```python
from build123d import *

# Parameters (mm, degrees)
SKETCH1_W                                = 152.4
SKETCH1_H                                = 101.6
BOSS_EXTRUDE1_DEPTH                      = 12.7
CBORE_FOR_3_8_HEX_HEAD_BOLT1_D           = 10.0838
CBORE_FOR_3_8_HEX_HEAD_BOLT1_CBORE_D     = 15.24
CBORE_FOR_3_8_HEX_HEAD_BOLT1_CBORE_DEPTH = 11.176
TAP_DRILL_FOR_1_4_20_TAP1_D              = 5.1054


with BuildPart() as part:
    # Sketch1 → Boss-Extrude1 (new body)
    with BuildSketch(Plane(origin=(0, 0, 0), x_dir=(1, 0, 0), z_dir=(0, 1, 0))):
        Rectangle(SKETCH1_W, SKETCH1_H)
    extrude(amount=BOSS_EXTRUDE1_DEPTH)

    # CBORE for 3/8 Hex Head Bolt1 (through all)
    with Locations(Plane(origin=(0, 12.7, 0), x_dir=(1, 0, 0), z_dir=(0, 1, 0))):
        with Locations((-50.000000076, 0), (50.000000076, 0), (0, 0)):
            CounterBoreHole(CBORE_FOR_3_8_HEX_HEAD_BOLT1_D / 2, CBORE_FOR_3_8_HEX_HEAD_BOLT1_CBORE_D / 2, CBORE_FOR_3_8_HEX_HEAD_BOLT1_CBORE_DEPTH)

    # Tap Drill for 1/4-20 Tap1 (through all)
    with Locations(Plane.XZ):
        with Locations((-38.1, -38.1), (38.1, -38.1), (38.1, 38.1), (-38.1, 38.1)):
            Hole(TAP_DRILL_FOR_1_4_20_TAP1_D / 2)


solid = part.part
```
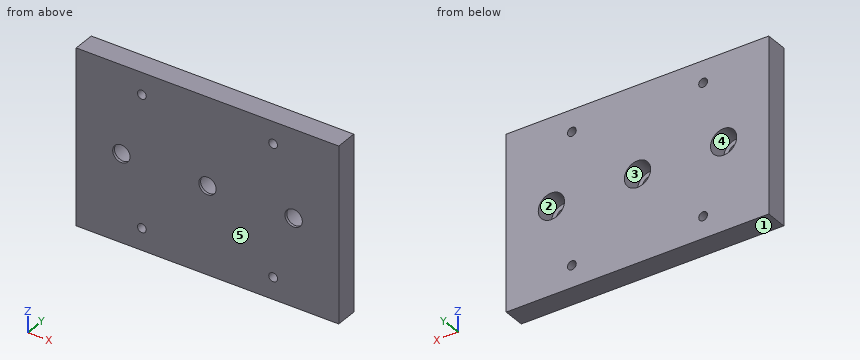
Geometry check sheet. Reference: the model listing, model coordinates, mm. Face numbers are marked on the shaded views. A direction names the side the tool comes from. Give positions to 0.01 mm unless a question says otherwise; leave off trailing zeros. Order: outer loops, then holes, each group sorted by start corner. A loop starts at its lowest first (then second) coordinate and runs counter-clockwise, first axis right, second up. Notation, with made-up numbers: (-2, 46) -> (46, 46) arc R12 cw to (46, 66) -> close; hole circle Ø4 at (21, -1). An arc over 180 degrees is marked (long way). Write each question's results on one line, items separated by ' | '. Start each with the question number.
(1) Sectioned sample at A-A (x = 38.1). Enter the section's corners in (y, z), plus the area to 3 significant figures.
(2) Sectioned sample at C-C (x = -50). Enter the section's corners in (y, z).
(3) Scan lines: line 1 (Z direction, x = -38.1, y = 4.75); line 2 (Z direction, x = -50, y = 0.95); line 3 (X direction, y = 6, z = -3). Record each from-to range of solid material in increasing order.
(4) Sectioned sample at B-B (z = 0). Enter the section's corners in (x, y), plus the area to 3 significant figures.
(5) Sectioned sample at D-D (y = 7.75). Enter the section's corners in (x, z).
(6) Mould release check, pull along X, two halves, no side actions. Record for the marked faces 1, 2 and 3: pulls with the +X half, pulls with the -X half, needs draft (parallel to the pull), parting line crosses it, or undercut.
(7) Gauge pin test, flat ends, axial feed: P1, Ø11.5, axis at x = 50, z = 0, coming from the +Y side; P2, Ø6, axis at x = -50, z = 0, coming from the -Y side. Record the tip position at first contact, or that the pin passes through.
(8) Access from +Z, -Z, +X, -X, +Y, -Y to the whole of each face (thin tool, end or side, straight path). Record for the marked faces 4 and 5.
Answer below:
1) outline: (0, -50.8) -> (12.7, -50.8) -> (12.7, -40.65) -> (0, -40.65) -> close; (0, -35.55) -> (12.7, -35.55) -> (12.7, 35.55) -> (0, 35.55) -> close; (0, 40.65) -> (12.7, 40.65) -> (12.7, 50.8) -> (0, 50.8) -> close | area: 1,160 mm2
2) outline: (0, -50.8) -> (12.7, -50.8) -> (12.7, -7.62) -> (1.52, -7.62) -> (1.52, -5.04) -> (0, -5.04) -> close; (0, 5.04) -> (1.52, 5.04) -> (1.52, 7.62) -> (12.7, 7.62) -> (12.7, 50.8) -> (0, 50.8) -> close
3) line 1: -50.8 to -40.65, -35.55 to 35.55, 40.65 to 50.8 | line 2: -50.8 to -5.04, 5.04 to 50.8 | line 3: -76.2 to -57, -43 to -7, 7 to 43, 57 to 76.2
4) outline: (-76.2, 0) -> (-55.04, 0) -> (-55.04, 1.52) -> (-57.62, 1.52) -> (-57.62, 12.7) -> (-76.2, 12.7) -> close; (-44.96, 0) -> (-5.04, 0) -> (-5.04, 1.52) -> (-7.62, 1.52) -> (-7.62, 12.7) -> (-42.38, 12.7) -> (-42.38, 1.52) -> (-44.96, 1.52) -> close; (5.04, 0) -> (44.96, 0) -> (44.96, 1.52) -> (42.38, 1.52) -> (42.38, 12.7) -> (7.62, 12.7) -> (7.62, 1.52) -> (5.04, 1.52) -> close; (55.04, 0) -> (76.2, 0) -> (76.2, 12.7) -> (57.62, 12.7) -> (57.62, 1.52) -> (55.04, 1.52) -> close | area: 1,380 mm2
5) outline: (-76.2, -50.8) -> (76.2, -50.8) -> (76.2, 50.8) -> (-76.2, 50.8) -> close; hole circle Ø15.24 at (-50, 0); hole circle Ø5.11 at (-38.1, -38.1); hole circle Ø5.11 at (-38.1, 38.1); hole circle Ø15.24 at (0, 0); hole circle Ø5.11 at (38.1, -38.1); hole circle Ø5.11 at (38.1, 38.1); hole circle Ø15.24 at (50, 0)
6) face 1: needs draft | face 2: undercut | face 3: undercut
7) P1: y = 1.52 | P2: through
8) face 4: +Y | face 5: +Z, -Z, +X, -X, -Y
